from build123d import *

# Parameters (mm, degrees)
SKETCH1_R           = 1.6
BOSS_EXTRUDE1_DEPTH = 52
CUT_EXTRUDE1_DEPTH  = 46
CUT_EXTRUDE2_DEPTH  = 3.6
CHAMFER1_SIZE       = 3
CHAMFER2_SIZE       = 0.5
BOSS_EXTRUDE2_DEPTH = 2
CHAMFER3_SIZE       = 1.5
CUT_EXTRUDE4_DEPTH  = 2.5


with BuildPart() as part:
    # Sketch1 → Boss-Extrude1 (new body)
    with BuildSketch(Plane.XY):
        with BuildLine():
            Line((-4.46161756, 0), (-3.2, 0))
            ThreePointArc((-3.2, 0), (-1.084064892, -3.010781179), (2.465502069, -2.039926359))
            Line((2.465502069, -2.039926359), (17.709814498, -14.652884646))
            ThreePointArc((17.709814498, -14.652884646), (19.682532968, -15.386676734), (21.68432718, -14.736377626))
            ThreePointArc((21.68432718, -14.736377626), (20.423085706, 15.613531633), (-7.590844762, 3.869281046))
            ThreePointArc((-7.590844762, 3.869281046), (-6.949759371, 1.187749934), (-4.46161756, 0))
        make_face()
        with Locations(Location((19.749740857, -12.187382577, 0), (0, 0, 180))):
            Circle(SKETCH1_R, mode=Mode.SUBTRACT)
        with Locations(Location((0, 0, 0), (0, 0, 180))):
            Circle(SKETCH1_R, mode=Mode.SUBTRACT)
    extrude(amount=BOSS_EXTRUDE1_DEPTH)

    # Sketch2 → Cut-Extrude1 (cut)
    with BuildSketch(Plane.XY.offset(52)):
        with BuildLine():
            Line((-7.75220957, 2.930270623), (-10.26732185, 3.33405514))
            ThreePointArc((-10.26732185, 3.33405514), (2.118916828, -19.291319949), (27.109557142, -12.904270303))
            Line((27.109557142, -12.904270303), (25.097988128, -11.341445354))
            ThreePointArc((25.097988128, -11.341445354), (23.677045606, -11.352651842), (23.546148123, -9.937706936))
            ThreePointArc((23.546148123, -9.937706936), (17.03488015, 15.04178651), (-5.667119596, 2.753950614))
            ThreePointArc((-5.667119596, 2.753950614), (-6.790684219, 1.884004769), (-7.75220957, 2.930270623))
        make_face()
    extrude(amount=-CUT_EXTRUDE1_DEPTH, mode=Mode.SUBTRACT)

    # Sketch3 → Cut-Extrude2 (cut)
    with BuildSketch(Plane.XY.offset(6)):
        with BuildLine():
            Line((1.692106757, 2.716021856), (20.436641856, -8.961997016))
            ThreePointArc((20.436641856, -8.961997016), (22.952539617, -9.338121402), (24.947839186, -7.760150957))
            ThreePointArc((24.947839186, -7.760150957), (18.297055064, 14.427956624), (-3.907979798, 7.833908229))
            ThreePointArc((-3.907979798, 7.833908229), (-3.696429412, 4.43953433), (-0.548333333, 3.152670385))
            ThreePointArc((-0.548333333, 3.152670385), (0.612143689, 3.140904345), (1.692106757, 2.716021856))
        make_face()
    extrude(amount=-CUT_EXTRUDE2_DEPTH, mode=Mode.SUBTRACT)

    # Chamfer1
    chamfer1_edges = [part.edges().sort_by_distance(p)[0] for p in [
        (0.612143689, 3.140904345, 2.4),
        (11.064374306, -3.12298758, 2.4),
        (22.952539617, -9.338121402, 2.4),
        (18.297055064, 14.427956624, 2.4),
        (-3.696429412, 4.43953433, 2.4),
    ]]
    chamfer(chamfer1_edges, length=CHAMFER1_SIZE)

    # Chamfer2
    chamfer2_edges = [part.edges().sort_by_distance(p)[0] for p in [
        (21.349740857, -12.187382577, 0),
        (1.6, 0, 0),
        (20.423085706, 15.613531633, 0),
        (19.682532968, -15.386676734, 0),
        (10.087658283, -8.346405502, 0),
        (-1.084064892, -3.010781179, 0),
        (-3.83080878, 0, 0),
        (-6.949759371, 1.187749934, 0),
    ]]
    chamfer(chamfer2_edges, length=CHAMFER2_SIZE)

    # Sketch4 → Boss-Extrude2 (add)
    with BuildSketch(Plane.XY.offset(52)):
        with BuildLine():
            Line((-6.147708238, 8.068693229), (-5.275417078, 9.868445471))
            ThreePointArc((-5.275417078, 9.868445471), (19.440984389, 18.44746048), (28.019999398, -6.268940987))
            Line((28.019999398, -6.268940987), (27.147708238, -8.068693229))
            Line((27.147708238, -8.068693229), (25.257968384, -7.152787511))
            ThreePointArc((25.257968384, -7.152787511), (17.652787511, 14.757968384), (-4.257968384, 7.152787511))
            Line((-4.257968384, 7.152787511), (-6.147708238, 8.068693229))
        make_face()
    extrude(amount=-BOSS_EXTRUDE2_DEPTH)

    # Chamfer3
    # the kernel refuses this chamfer: 1.5 mm, written as the material it takes off along each edge
    with BuildSketch(Plane(origin=(-7.83015049, 4.597399062, 50), x_dir=(0.8995358930200849, -0.43598068069350693, -0.02749587661058679), z_dir=(0.4361455799615031, 0.8998761209633491, 0))) as chamfer3_piece_1_section:
        Polygon((CHAMFER3_SIZE * 0.999621916911, -CHAMFER3_SIZE * 0.0274958766106), (-CHAMFER3_SIZE * 0.0274958766106, -CHAMFER3_SIZE * 0.999621916911), (0, 0), align=None)
    chamfer3_piece_1 = extrude(amount=5.857524482, mode=Mode.PRIVATE)
    chamfer3_piece_1 = chamfer3_piece_1 - Plane(origin=(10.5, 0, 50.729873863), x_dir=(0.6045582259252599, -0.7965609527626261, 0), z_dir=(0, 0, -1)) * Cylinder(18.5, 18, mode=Mode.PRIVATE)
    add(chamfer3_piece_1, mode=Mode.SUBTRACT)
    with BuildSketch(Plane(origin=(11.37229116, 1.799752242, 50), x_dir=(-0.899876120963349, 0.43614557996150355, 0), z_dir=(-0.43614557996150355, -0.899876120963349, 0))) as chamfer3_piece_2_section:
        Polygon((18.5, -CHAMFER3_SIZE), (18.5 - CHAMFER3_SIZE, 0), (18.5, 0), align=None)
    chamfer3_piece_2 = revolve(axis=Axis((11.37229116, 1.799752242, 50), (0, 0, -1)), revolution_arc=180, mode=Mode.PRIVATE)
    chamfer3_piece_2 = chamfer3_piece_2 - Plane(origin=(10.5, 0, 50.723063531), x_dir=(0.6045582259252599, -0.7965609527626261, 0), z_dir=(0, 0, -1)) * Cylinder(18.5, 75, mode=Mode.PRIVATE)
    add(chamfer3_piece_2, mode=Mode.SUBTRACT)
    with BuildSketch(Plane(origin=(28.019999398, -6.268940987, 50), x_dir=(0.024742882786820786, -0.011992205050873842, 0.9996219169112968), z_dir=(-0.43614557996150277, -0.8998761209633493, 0))) as chamfer3_piece_3_section:
        Polygon((CHAMFER3_SIZE * 0.999621916911, CHAMFER3_SIZE * 0.0274958766106), (-CHAMFER3_SIZE * 0.0274958766106, CHAMFER3_SIZE * 0.999621916911), (0, 0), align=None)
    chamfer3_piece_3 = extrude(amount=5.857524482, mode=Mode.PRIVATE)
    chamfer3_piece_3 = chamfer3_piece_3 - Plane(origin=(10.5, 0, 50.745956447), x_dir=(0.6045582259252599, -0.7965609527626261, 0), z_dir=(0, 0, -1)) * Cylinder(18.5, 18, mode=Mode.PRIVATE)
    add(chamfer3_piece_3, mode=Mode.SUBTRACT)

    # Sketch5 → Cut-Extrude4 (cut)
    with BuildSketch(Plane.XY.offset(6)):
        Polygon((3.348631561, 0), (1.674315781, 2.9), (-1.674315781, 2.9), (-5.480163243, -3.691921171), (0.106662744, -5.615254708), align=None)
        Polygon((18.075425076, -9.287382577), (13.043037161, -18.003734129), (26.456444552, -18.003734129), (21.424056637, -9.287382577), align=None)
    extrude(amount=-CUT_EXTRUDE4_DEPTH, mode=Mode.SUBTRACT)


solid = part.part
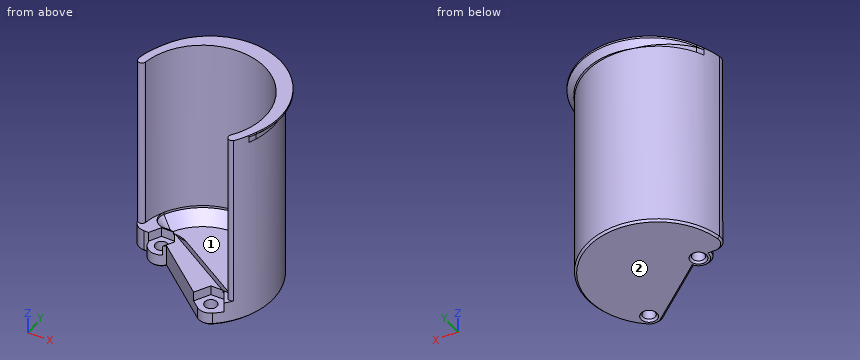
The model under review builds one solid part; all positions refer to its coordinate system, in mm. Face numbers are marked on the shaded views. Coordinates: 2 decimals unless noted, no trailing zeros. Put each result on its own line as item: value.
1) Draft analysis for pull direction X (two halves, no side actions). For the marked faces 1 and 2, state which applies: released by +X, released by -X, zero draft, split by the parting line, or undercut.
Computed:
face 1: undercut
face 2: zero draft
2) Wall thickness on probe 1 along Y at (x, z) = (10.5, 20); probe 2 along X at (y, z) = (7, 39.5); probe 3 along X at (y, z) = (5.5, 8): over which ranges is each line inside the solid? List them lowest first. Write a range as [from, to].
Computed:
probe 1: y = [16.4, 18.5]
probe 2: x = [-6.62, -4.33], [25.33, 27.62]
probe 3: x = [-7.16, -4.95], [25.95, 28.16]
3) Clearance check with flat-ended pins moving along their axes: pin 1 Ø1.5 at (x, z) = (25, 36) entering from +Y; pin 2 Ø1 at (y, z) = (-5, 33) entering from +X; pin 3 Ø4.5 at (x, y) = (8, -8.5) entering from +Z. State where each tip first meets the part, or that it passes through.
Computed:
pin 1: stops at y = 12.38
pin 2: stops at x = 28.44
pin 3: stops at z = 6
